Check sheet for the modelled part. Datum: model origin and axes. Units: mm. A direction names the side the tool comes from. Give positions to 0.01 mm unless a question says otherwise; leave off trailing zeros. Order: outer loops, then holes, each group sorted by start corner. A loop starts at its lowest first (then second) coordinate and runs counter-clockwise, first axis right, second up.
Item 1: Access from +Z, -Z, +X, -X, +Y, -Y to the whole of each face (thin tool, end or side, straight path). Record for faces 4 (the flat face through (200.3, 228.6, 35.4)), 5 (the flat face through (-62.523, -8, -61)), 6 (the flat face through (363, 100, -263.451)), 7 (the flat face through (102.577, 113, 41)), 8 (the flat face through (279, 113, 47.699)).
Item 2: Sectioned sample at A-A on z = -312. Record the boundary of the cut face in (x, y).
Item 3: Sectioned sample at C-C on x = 263. Record the boundary of the cut face in (y, z).
Item 4: Sectioned sample at B-B on y = 144. Record the boundary of the cut face in (x, z).
Item 5: Release check for a two-part mould opening along Y. For faces 1 (the flat face through (356.577, 113, -112)), 2 (the flat face through (363, 203.2, -317)), 3 (the flat face through (150, -12.7, -152)) record: released by +Y, released by -Y, zero draft, split by the parting line, or undercut.
Item 6: Sectioned sample at D-D on z = -174.5. Record the boundary of the cut face in (x, y).
Item 7: Material ranges on line 1 along Y through (x, z) = (300.5, -275.5); line 2 along X through (y, z) = (169, -6); line 3 along Z through (x, y) = (316.5, 170), recorded low to high.
Item 8: Gauge pin test, flat ends, axial feed: P1, Ø6, axis at x = 179.5, y = 137, coming from the -Z side; P2, Ø12, axis at y = 201, z = -246, coming from the -X side; P3, Ø14, axis at x = 362.5, y = 80, coming from the -Z side. Record the tip position at first contact, or that the pin passes through.
from build123d import *

# Parameters (mm, degrees)
SKETCH1_W           = 431.8
SKETCH1_H           = 431.8
SKETCH1_W_2         = 406.4
SKETCH1_H_2         = 406.4
EXTRUDE_THIN1_DEPTH = 228.6
SKETCH2_W           = 431.8
SKETCH2_H           = 431.8
EXTRUDE1_DEPTH      = 12.7
CUT_EXTRUDE1_DEPTH  = 229.6
EXTRUDE2_DEPTH      = 228.6
SKETCH5_W           = 12.7
SKETCH5_H           = 107.95
CUT_EXTRUDE2_DEPTH  = 203.2


with BuildPart() as part:
    # Sketch1 → Extrude-Thin1 (new body)
    with BuildSketch(Plane(origin=(0, 0, 0), x_dir=(1, 0, 0), z_dir=(0, 1, 0))):
        with Locations((153.377464009, 155.501162791)):
            Rectangle(SKETCH1_W, SKETCH1_H)
        with Locations((153.377464009, 155.501162791)):
            Rectangle(SKETCH1_W_2, SKETCH1_H_2, mode=Mode.SUBTRACT)
    extrude(amount=EXTRUDE_THIN1_DEPTH)

    # Sketch2 → Extrude1 (add)
    with BuildSketch(Plane.XZ):
        with Locations((153.377464009, -155.501162791)):
            Rectangle(SKETCH2_W, SKETCH2_H)
    extrude(amount=EXTRUDE1_DEPTH)

    # Sketch3 → Cut-Extrude1 (cut, through all)
    with BuildSketch(Plane(origin=(0, 0, 0), x_dir=(-1, 0, 0), z_dir=(0, 1, 0))):
        Polygon((-356.577464009, -371.401162791), (62.522535991, -371.401162791), (62.522535991, 47.698837209), (49.822535991, 47.698837209), (49.822535991, -358.701162791), (-356.577464009, -358.701162791), align=None)
    extrude(amount=CUT_EXTRUDE1_DEPTH, mode=Mode.SUBTRACT)

    # Sketch4 → Extrude2 (add)
    with BuildSketch(Plane(origin=(0, 0, 0), x_dir=(-1, 0, 0), z_dir=(0, 1, 0))):
        Polygon((-153.377464009, 60.398837209), (-204.177464009, 60.398837209), (-204.177464009, 34.998837209), (-153.377464009, 34.998837209), (-102.577464009, 34.998837209), (-102.577464009, 60.398837209), align=None)
    extrude(amount=EXTRUDE2_DEPTH)

    # Sketch5 → Cut-Extrude2 (cut)
    with BuildSketch(Plane(origin=(0, 0, 0), x_dir=(-1, 0, 0), z_dir=(0, 1, 0))):
        with Locations((-362.927464009, -317.426162791)):
            Rectangle(SKETCH5_W, SKETCH5_H)
    extrude(amount=CUT_EXTRUDE2_DEPTH, mode=Mode.SUBTRACT)


solid = part.part
Report:
1. face 4: +Z, -Z, +X, -X, +Y
1. face 5: +Z, -Z, -X, +Y, -Y
1. face 6: -Z, +X, -X
1. face 7: -Z, -X, +Y
1. face 8: -Z, +Y
2. outline: (-62.52, -12.7) - (369.28, -12.7) - (369.28, 0) - (-62.52, 0) - close; (356.58, 203.2) - (369.28, 203.2) - (369.28, 228.6) - (356.58, 228.6) - close
3. outline: (-12.7, -371.4) - (0, -371.4) - (0, 47.7) - (228.6, 47.7) - (228.6, 60.4) - (-12.7, 60.4) - close
4. outline: (-62.52, 47.7) - (102.58, 47.7) - (102.58, 35) - (204.18, 35) - (204.18, 47.7) - (356.58, 47.7) - (356.58, -263.45) - (369.28, -263.45) - (369.28, 60.4) - (-62.52, 60.4) - close
5. face 1: zero draft
5. face 2: undercut
5. face 3: released by -Y
6. outline: (-62.52, -12.7) - (369.28, -12.7) - (369.28, 228.6) - (356.58, 228.6) - (356.58, 0) - (-62.52, 0) - close
7. line 1: y = -12.7 to 0
7. line 2: x = 356.58 to 369.28
7. line 3: z = 47.7 to 60.4
8. P1: stops at z = 35
8. P2: stops at x = 356.58
8. P3: stops at z = -263.45
